The model under review builds one solid part; all positions refer to its coordinate system, in mm. A direction names the side the tool comes from. Coordinates: 2 decimals unless noted, no trailing zeros. Order: outer loops, then holes, each group sorted by start corner. A loop starts at its lowest first (then second) coordinate and runs counter-clockwise, first axis right, second up. Notation, with made-up numbers: M -17,15.25 L 17,15.25 A35 cw 17,49.25 Z; hole C -13,68 d3. An arc over 180 degrees is marked long. One line per item, written item: value.
```python
from build123d import *

# Parameters (mm, degrees)
F0_W     = 12
F0_H     = 15
F0_R     = 4.25
F1_DEPTH = 24
F2_R     = 4.125
F2_R_2   = 4.25
F3_DEPTH = 2.8
F5_W     = 22.825278
F5_H     = 44.441271
F6_DEPTH = 25


with BuildPart() as f1:
    # F0 (on Front) → F1 (new body)
    with BuildSketch(Plane.XZ):
        Rectangle(F0_W, F0_H)
        with Locations((0, -1)):
            Circle(F0_R, mode=Mode.SUBTRACT)
    extrude(amount=F1_DEPTH)

    # F2 (on face) → F3 (cut)
    with BuildSketch(Plane.XY.offset(7.5)):
        with Locations((0, -6)):
            Circle(F2_R)
        with Locations((0, -17)):
            Circle(F2_R_2)
    extrude(amount=-F3_DEPTH, mode=Mode.SUBTRACT)

    # F5 (on offset) → F6 (cut)
    with BuildSketch(Plane.XZ.offset(11)):
        with Locations((0.147067, 4.025047)):
            Rectangle(F5_W, F5_H)
    extrude(amount=-F6_DEPTH, mode=Mode.SUBTRACT)


solid = f1.part
```
(1) Insertion check: pin 1 Ø4 at (x, y) = (1, -16) entering from +Z. The pin has a flat end and moves straight along its axis. Give the tip position at first contact, or say it passes through.
Geometry results:
pin 1: stops at z = 4.7
(2) For L1, parallel to X at y = -15, z = -1; L2, parallel to Y at x = 0, z = 5.95; L3, parallel to Z at x = 0, y = -18.75, list the stretches that pass through material, from the lowest coordinate up.
Geometry results:
L1: x = -6 to -4.25, 4.25 to 6
L2: y = -24 to -21.25, -12.75 to -11
L3: z = -7.5 to -5.25, 3.25 to 4.7
(3) Mouldability with a two-part tool opening along X and no side actions: class faces 3 (the flat face through (-6, -17, 0)), 4 (the flat face through (0, -22, 7.5)), 5 (the cylindrical face through (-0.92, -17.41, -5.15)) as +X half, -X half, draft (parallel to the pull), parting line (faces both ways), or undercut.
Geometry results:
face 3: -X half
face 4: draft
face 5: undercut
(4) We need section B-B, the plane z = -1. State the section outline as (x, y) points, plus the area to 3 significant figures.
Geometry results:
outline: M -6,-24 L -4.25,-24 L -4.25,-11 L -6,-11 Z; M 4.25,-24 L 6,-24 L 6,-11 L 4.25,-11 Z
area: 45.5 mm2
(5) We need section A-A, the plane x = -2. State the section outline as (y, z) points.
Geometry results:
outline: M -24,-7.5 L -11,-7.5 L -11,-4.75 L -24,-4.75 Z; M -24,2.75 L -11,2.75 L -11,7.5 L -13.25,7.5 L -13.25,4.7 L -20.75,4.7 L -20.75,7.5 L -24,7.5 Z
(6) We need section D-D, the plane z = 5.5. State the section outline as (x, y) points, plus the area to 3 significant figures.
Geometry results:
outline: M -6,-24 L 6,-24 L 6,-11 L -6,-11 Z; hole C 0,-17 d8.5
area: 99.3 mm2
(7) We need section C-C, the plane y = -19. State the section outline as (x, z) points.
Geometry results:
outline: M -6,-7.5 L 6,-7.5 L 6,7.5 L 3.75,7.5 L 3.75,4.7 L -3.75,4.7 L -3.75,7.5 L -6,7.5 Z; hole C 0,-1 d8.5
(8) Tool access review of faces 1 (the flat face through (6, -17, 0)), 2 (the flat face through (0, -17, 4.7)): name each direction out of +Z, -Z, +X, -X, +Y, -Y from which nothing blocks a thin tool from reaching the whole face with its end or side.
Geometry results:
face 1: +Z, -Z, +X, +Y, -Y
face 2: +Z
